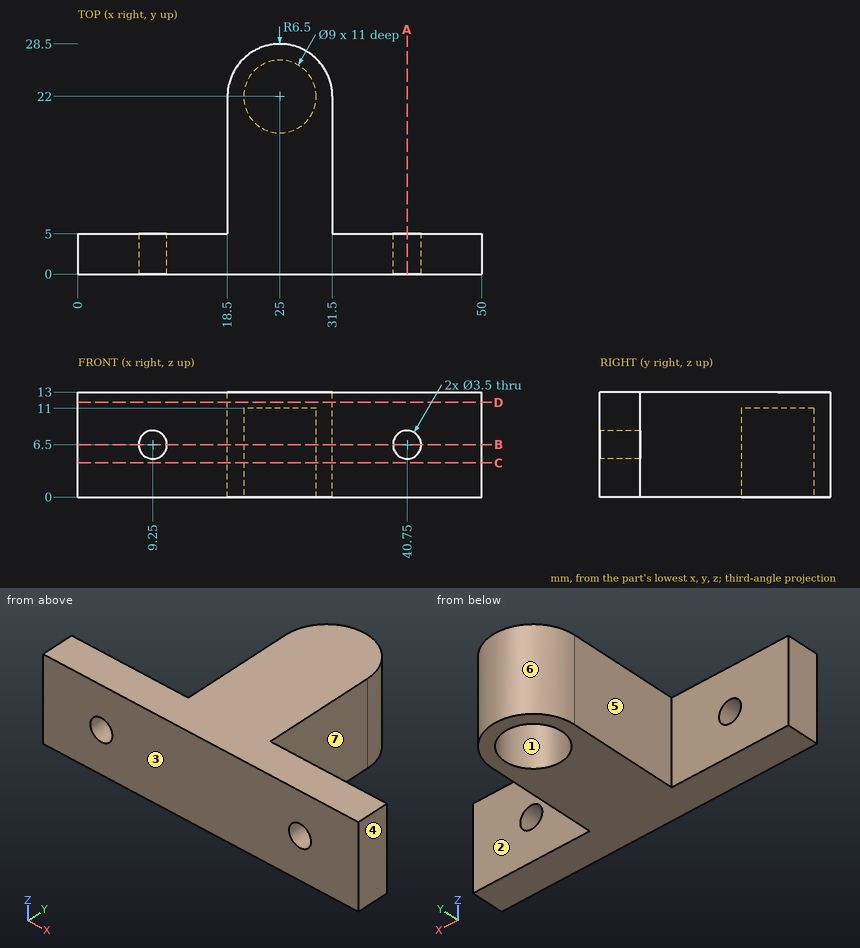
Could you check a few things on this drawing? It's one solid part, dimensions in mm from its lowest x, y, z. A direction names the side the tool comes from. Coordinates: 2 decimals unless noted, no trailing zeros. Order: outer loops, then holes, each group sorted by start corner. A loop starts at its lowest first (then second) coordinate and runs counter-clockwise, first axis right, second up.
1) Imagine slicing it at A-A on x = 40.75. List the corners of the cut face in (y, z) for me, and give its area (3 significant figures).
2) Which directions (+Z, -Z, +X, -X, +Y, -Y) give clear straight access to the entire face, cutting with the end or side of a thin tool? Please do the marked faces 5, 6 and 7.
3) Will these pins go through, and if not, where does the flat tip stop? pin 1 (1 mm diameter, centred on y = 17.5, z = 6, fed in from -X); pin 2 (4 mm diameter, centred on y = 18, z = 8, fed in from +X); pin 3 (6 mm diameter, centred on x = 8, z = 8, fed in from -Y); pin 4 (6.5 mm diameter, centred on x = 45, z = 4.5, fed in from +Y).
4) I need wall thicknesses on line 1 (Y direction, x = 25, z = 5); line 2 (Z direction, x = 9.25, y = 1.8); line 3 (X direction, y = 15.75, z = 12.5). Which ranges of each line are inside material? Lowest first, please.
5) Imagine slicing it at D-D on z = 11.75. List the corners of the cut face in (x, y) for me.
6) Imagine slicing it at C-C on z = 4.25. List the corners of the cut face in (x, y) for me, and give its area (3 significant figures).
7) We'd pull the mould along Y, two halves only. Please class the marked faces 1, 2, 3 and 4: +Y half, -Y half, draft (parallel to the pull), parting line (faces both ways), or undercut.
8) Imagine slicing it at B-B on z = 6.5. List the corners of the cut face in (x, y) for me, and give its area (3 significant figures).
Response values:
1. outline: (0, 0) - (5, 0) - (5, 4.75) - (0, 4.75) - close; (0, 8.25) - (5, 8.25) - (5, 13) - (0, 13) - close
1. area: 47.5 mm2
2. face 5: +Z, -Z, -X, +Y
2. face 6: +Z, -Z, +Y
2. face 7: +Z, -Z, +X, +Y
3. pin 1: stops at x = 18.5
3. pin 2: stops at x = 31.5
3. pin 3: stops at y = 0
3. pin 4: stops at y = 5
4. line 1: y = 0 to 17.5, 26.5 to 28.5
4. line 2: z = 0 to 4.75, 8.25 to 13
4. line 3: x = 18.5 to 31.5
5. outline: (0, 0) - (50, 0) - (50, 5) - (31.5, 5) - (31.5, 22) arc R6.5 ccw to (18.5, 22) - (18.5, 5) - (0, 5) - close
6. outline: (0, 0) - (50, 0) - (50, 5) - (31.5, 5) - (31.5, 22) arc R6.5 ccw to (18.5, 22) - (18.5, 5) - (0, 5) - close; hole circle Ø9 at (25, 22)
6. area: 474 mm2
7. face 1: undercut
7. face 2: +Y half
7. face 3: -Y half
7. face 4: draft
8. outline: (0, 0) - (7.5, 0) - (7.5, 5) - (0, 5) - close; (11, 0) - (39, 0) - (39, 5) - (31.5, 5) - (31.5, 22) arc R6.5 ccw to (18.5, 22) - (18.5, 5) - (11, 5) - close; (42.5, 0) - (50, 0) - (50, 5) - (42.5, 5) - close; hole circle Ø9 at (25, 22)
8. area: 439 mm2
